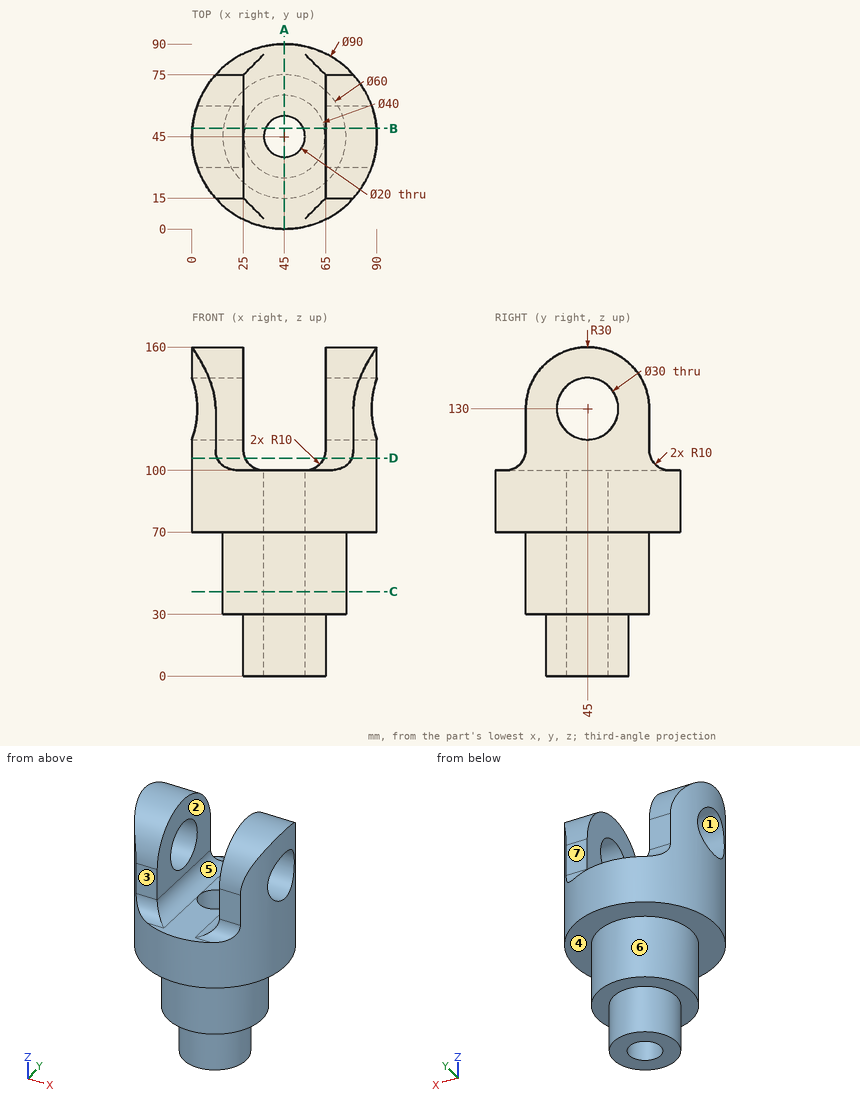
Can you work these out from the drawing? Everything is in mm from the part's minimum corner. A direction names the side the tool comes from. Round coordinates to 2 decimals unless told otherwise and drop trailing zeros. Order: outer loops, then holes, each group sorted by start corner. A loop starts at its lowest first (then second) coordinate and runs counter-clockwise, first axis right, second up. Notation, with made-up numbers: (-28.5, -26.75) -> (8.5, -26.75) arc R8 ccw to (8.5, -15.75) -> close; hole circle Ø5 at (-18, 86). An arc over 180 degrees is marked (long way). Return JSON: item names as keys, results as strings. Group by question number.
1. If we section it at D-D, the plane z = 106: Write out the boundary of the cut face in (x, y), then the cut area to 3 significant figures.
2. Which directions (+Z, -Z, +X, -X, +Y, -Y) give clear straight access to the entire face, cutting with the end or side of a thin tool? Please do the marked faces 1, 2, 3 and 4.
3. I need wall thicknesses on line 1 (Y direction, x = 12.5, z = 130); line 2 (Y direction, x = 45, z = 59); line 3 (Z direction, x = 39, y = 83). Which ranges of each line are inside material? Lowest first, please. Write a range as [from, to].
4. If we section it at B-B, the plane y = 49: Count the separate pieces of the cut face and the enclosed holes in it, then the cut area to 3 significant figures.
5. If we section it at C-C, the plane z = 41: Write out the boundary of the cut face in (x, y).
6. We'd pull the mould along X, two halves only. Please class the marked faces 5, 6 and 7: released by +X, released by -X, zero draft, split by the parting line, or undercut.
7. If we section it at A-A, the plane x = 45: Write out the boundary of the cut face in (y, z).
8. Will these pins go through, and if not, where does the flat tip stop? pin 1 (8 mm diameter, centred on y = 64, z = 71.5, fed in from +X); pin 2 (2 mm diameter, centred on x = 45, z = 35.5, fed in from -Y); pin 3 (1 mm diameter, centred on x = 74.5, y = 59.5, fed in from -Z).
Output values:
{
 "1": {"outline": "(12.22, 14.17) -> (25.83, 14.17) -> (25.83, 75.83) -> (12.22, 75.83) arc R45 ccw to start; (64.17, 14.17) -> (77.78, 14.17) arc R45 ccw to (77.78, 75.83) -> (64.17, 75.83) -> close", "area": "2,710 mm²"},
 "2": {"face 1": "+X, -X", "face 2": "+Z, +Y, -Y", "face 3": "+Z, +X, -X, -Y", "face 4": "-Z"},
 "3": {"line 1": "[15, 30], [60, 75]", "line 2": "[15, 35], [55, 75]", "line 3": "[70, 100]"},
 "4": {"separate pieces": "4", "enclosed holes": "0", "area": "5,980 mm²"},
 "5": {"outline": "circle Ø60 at (45, 45); hole circle Ø20 at (45, 45)"},
 "6": {"face 5": "undercut", "face 6": "split by the parting line", "face 7": "zero draft"},
 "7": {"outline": "(0, 70) -> (15, 70) -> (15, 30) -> (25, 30) -> (25, 0) -> (35, 0) -> (35, 100) -> (0, 100) -> close; (55, 0) -> (65, 0) -> (65, 30) -> (75, 30) -> (75, 70) -> (90, 70) -> (90, 100) -> (55, 100) -> close"},
 "8": {"pin 1": "x = 87.43", "pin 2": "y = 15", "pin 3": "z = 70"}
}
